Check sheet for the modelled part. Datum: model origin and axes. Units: mm. A direction names the side the tool comes from. Give positions to 0.01 mm unless a question says otherwise; leave off trailing zeros. Order: outer loops, then holes, each group sorted by start corner. A loop starts at its lowest first (then second) coordinate and runs counter-clockwise, first axis right, second up.
from build123d import *

# Parameters (mm, degrees)
CROQUIS1_R              = 3.75
CROQUIS1_R_2            = 1.65
SALIENTE_EXTRUIR1_DEPTH = 2
SALIENTE_EXTRUIR2_DEPTH = 2
CROQUIS5_R              = 1.5
CORTAR_EXTRUIR2_DEPTH   = 10
REDONDEO3_R             = 1
REDONDEO4_R             = 1
REDONDEO5_R             = 1
REDONDEO6_R             = 1
REDONDEO7_R             = 1
REDONDEO8_R             = 1
REDONDEO12_R            = 2


with BuildPart() as part:
    # Croquis1 → Saliente-Extruir1 (new body)
    with BuildSketch(Plane.XY):
        with BuildLine():
            Line((0, 0), (0, 25))
            Line((0, 25), (14.5, 25))
            ThreePointArc((14.5, 25), (27, 12.5), (14.5, 0))
            Line((14.5, 0), (0, 0))
        make_face()
        with Locations((14.5, 12.5)):
            Circle(CROQUIS1_R, mode=Mode.SUBTRACT)
        with Locations((14.5, 21)):
            Circle(CROQUIS1_R_2, mode=Mode.SUBTRACT)
        with Locations((23, 12.5)):
            Circle(CROQUIS1_R_2, mode=Mode.SUBTRACT)
        with Locations((14.5, 4)):
            Circle(CROQUIS1_R_2, mode=Mode.SUBTRACT)
        with Locations((6, 12.5)):
            Circle(CROQUIS1_R_2, mode=Mode.SUBTRACT)
    extrude(amount=SALIENTE_EXTRUIR1_DEPTH)

    # Croquis4 → Saliente-Extruir2 (add)
    with BuildSketch(Plane.ZY):
        with BuildLine():
            Line((2, 0), (-46.922808665, 0))
            ThreePointArc((-46.922808665, 0), (-48.234090069, 0.765909931), (-49, 2.077191335))
            Line((-49, 2.077191335), (-49, 22.665501207))
            ThreePointArc((-49, 22.665501207), (-48.183232344, 24.133251816), (-46.715481735, 24.950019472))
            Line((-46.715481735, 24.950019472), (2, 24.950019472))
            Line((2, 24.950019472), (2, 0))
        make_face()
    extrude(amount=-SALIENTE_EXTRUIR2_DEPTH)

    # Croquis5 → Cortar-Extruir2 (cut)
    with BuildSketch(Plane(origin=(2, 0, 0), x_dir=(0, 0, -1), z_dir=(1, 0, 0))):
        with Locations((44.4, 12.371346271)):
            Circle(CROQUIS5_R)
        with Locations((38.2, 12.371346271)):
            Circle(CROQUIS5_R)
        with Locations((32, 12.371346271)):
            Circle(CROQUIS5_R)
        with Locations((25.8, 12.371346271)):
            Circle(CROQUIS5_R)
        with Locations((19.6, 12.371346271)):
            Circle(CROQUIS5_R)
        with Locations((13.4, 12.371346271)):
            Circle(CROQUIS5_R)
        with Locations((7.2, 12.371346271)):
            Circle(CROQUIS5_R)
        with Locations((4.2, 24.5)):
            Circle(CROQUIS5_R)
        with Locations((10.4, 24.5)):
            Circle(CROQUIS5_R)
        with Locations((16.6, 24.5)):
            Circle(CROQUIS5_R)
        with Locations((22.8, 24.5)):
            Circle(CROQUIS5_R)
        with Locations((29, 24.5)):
            Circle(CROQUIS5_R)
        with Locations((35.2, 24.5)):
            Circle(CROQUIS5_R)
        with Locations((41.4, 24.5)):
            Circle(CROQUIS5_R)
        with Locations((41.4, 0.242692542)):
            Circle(CROQUIS5_R)
        with Locations((35.2, 0.242692542)):
            Circle(CROQUIS5_R)
        with Locations((29, 0.242692542)):
            Circle(CROQUIS5_R)
        with Locations((22.8, 0.242692542)):
            Circle(CROQUIS5_R)
        with Locations((16.6, 0.242692542)):
            Circle(CROQUIS5_R)
        with Locations((10.4, 0.242692542)):
            Circle(CROQUIS5_R)
        with Locations((4.2, 0.242692542)):
            Circle(CROQUIS5_R)
    extrude(amount=-CORTAR_EXTRUIR2_DEPTH, mode=Mode.SUBTRACT)

    # Redondeo3
    redondeo3_edges = [part.edges().sort_by_distance(p)[0] for p in [
        (1, 24.950019472, -5.630902678),
        (1, 24.950019472, -8.969097322),
    ]]
    fillet(redondeo3_edges, radius=REDONDEO3_R)

    # Redondeo4
    redondeo4_edges = [part.edges().sort_by_distance(p)[0] for p in [
        (1, 24.950019472, -21.369097322),
        (1, 24.950019472, -11.830902678),
        (1, 24.950019472, -15.169097322),
        (1, 24.950019472, -18.030902678),
    ]]
    fillet(redondeo4_edges, radius=REDONDEO4_R)

    # Redondeo5
    redondeo5_edges = [part.edges().sort_by_distance(p)[0] for p in [
        (1, 24.950019472, -39.969097322),
        (1, 24.950019472, -42.830902678),
        (1, 24.950019472, -33.769097322),
        (1, 24.950019472, -36.630902678),
        (1, 24.950019472, -27.569097322),
        (1, 24.950019472, -30.430902678),
        (1, 24.950019472, -24.230902678),
    ]]
    fillet(redondeo5_edges, radius=REDONDEO5_R)

    # Redondeo6
    redondeo6_edges = [part.edges().sort_by_distance(p)[0] for p in [
        (1, 24.950019472, -2.769097322),
    ]]
    fillet(redondeo6_edges, radius=REDONDEO6_R)

    # Redondeo7
    redondeo7_edges = [part.edges().sort_by_distance(p)[0] for p in [
        (1, 0, -27.519763421),
        (1, 0, -21.319763421),
        (1, 0, -24.280236579),
        (1, 0, -15.119763421),
        (1, 0, -18.080236579),
        (1, 0, -8.919763421),
        (1, 0, -11.880236579),
        (1, 0, -2.719763421),
        (1, 0, -5.680236579),
    ]]
    fillet(redondeo7_edges, radius=REDONDEO7_R)

    # Redondeo8
    redondeo8_edges = [part.edges().sort_by_distance(p)[0] for p in [
        (1, 0, -33.719763421),
        (1, 0, -36.680236579),
        (1, 0, -39.919763421),
        (1, 0, -42.880236579),
        (1, 0, -30.480236579),
    ]]
    fillet(redondeo8_edges, radius=REDONDEO8_R)

    # Redondeo12
    redondeo12_edges = [part.edges().sort_by_distance(p)[0] for p in [
        (0, 12.5, 2),
    ]]
    fillet(redondeo12_edges, radius=REDONDEO12_R)


solid = part.part
1) Material ranges on L1, parallel to Y at x = 14.5, z = 1.25; L2, parallel to Y at x = 1.05, z = -44.4; L3, parallel to Z at x = 3.25, y = 6.25, recorded low to high.
Recorded:
L1: y = 0 to 2.35, 5.65 to 8.75, 16.25 to 19.35, 22.65 to 25
L2: y = 0 to 10.87, 13.87 to 24.95
L3: z = 0 to 2
2) Draft check along Z on faces 4 (the face through (1.014, 11.797, -45.786)), 5 (the face through (7, 25, 1)). Enter one of: +Z half, -Z half, draft (parallel to the pull), parting line (faces both ways), or undercut.
Recorded:
face 4: undercut
face 5: draft
3) Section check B-B, the plane y = 4. Record the cut outline in (x, z), then the cut area to 3 significant figures.
Recorded:
outline: (0, -49) - (2, -49) - (2, 0) - (12.85, 0) - (12.85, 2) - (2, 2) arc R2 ccw to (0, 0) - close; (16.15, 0) - (23.67, 0) - (23.67, 2) - (16.15, 2) - close
area: 138 mm2
4) Depth check by flat-ended pin: pin 1 Ø12 at (x, y) = (14.5, 12.5) entering from -Z; pin 2 Ø1.5 at (x, z) = (4.5, -33) entering from -Y (3 decimals); pin 3 Ø8 at (y, z) = (4.5, -13.5) entering from +X; pin 4 Ø4 at (x, z) = (3, -38) entering from +Y. Enter the tip coordinate at first touch or a pass-through.
Recorded:
pin 1: stops at z = 0
pin 2: passes through
pin 3: stops at x = 2
pin 4: stops at y = 24.95
5) Section check C-C, the plane z = -13.4. Record the cut outline in (x, y).
Recorded:
outline: (0, 0) - (2, 0) - (2, 10.87) - (0, 10.87) - close; (0, 13.87) - (2, 13.87) - (2, 24.95) - (0, 24.95) - close
6) Set-up check for faces 1 (the face through (1.014, 0.198, -12.185)), 2 (the face through (1.014, 24.737, -14.778)), 3 (the face through (1, 12.4, -18.1)): record each of +Z, -Z, +X, -X, +Y, -Y from which the full face is reachable in a straight line by a thin tool's end or side.
Recorded:
face 1: +X, -X, -Y
face 2: +X, -X, +Y
face 3: +X, -X
7) Section check A-A, the plane x = 6. Record the cut outline in (y, z), then the cut area to 3 significant figures.
Recorded:
outline: (0, 0) - (10.85, 0) - (10.85, 2) - (0, 2) - close; (14.15, 0) - (25, 0) - (25, 2) - (14.15, 2) - close
area: 43.4 mm2
8) Section check D-D, the plane y = 18.75. Record the cut outline in (x, z), then the cut area to 3 significant figures.
Recorded:
outline: (0, -49) - (2, -49) - (2, 0) - (25.33, 0) - (25.33, 2) - (2, 2) arc R2 ccw to (0, 0) - close
area: 148 mm2
